from build123d import *

# Parameters (mm, degrees)
F0_R     = 11.65
F0_R_2   = 11
F1_DEPTH = 180
F3_DEPTH = 0.4
F4_COUNT = 8


with BuildPart() as f1:
    # F0 (on Front) → F1 (new body)
    with BuildSketch(Plane.XZ):
        Circle(F0_R)
        Circle(F0_R_2, mode=Mode.SUBTRACT)
    extrude(amount=F1_DEPTH)

    # F2 (on Top) → F3 (join, symmetric)
    with BuildSketch(Plane.XY):
        Polygon((-11.318761, -35.867412), (-11.318761, 0), (-23.984207, 0), (-23.984207, -22.375958), align=None)
    extrude(amount=F3_DEPTH, both=True)

    # F4: F1 ×8 about axis
    f4_axis = Axis((0, 0, 0), (0, 1, 0))


with BuildPart() as f1_1:
    add(f1.part)
    for i in range(1, F4_COUNT):
        add(f1.part.rotate(f4_axis, i * 360 / F4_COUNT))


solid = f1_1.part
Geometry: final body of the model. Coordinates: model frame, mm. A direction names the side the tool comes from. Give positions to 0.01 mm unless a question says otherwise; leave off trailing zeros. Write each loop counter-clockwise with the first axis right and the second up, starting at its lowest first coordinate (ties: lowest second). Pieces come first, ordered by that corner, then holes.
(1) Cut plane D-D, the plane x = 13.5. Return loops of the section in (y, z), then the cut area to 3 significant figures.
(2) Ray query, line 1 (Z direction, x = 0, y = -127); line 2 (X direction, y = -15, z = -12.5); line 3 (X direction, y = -10.5, z = -10). Return the intervals inside material, ascending.
(3) Cut plane A-A, the plane z = 14. Return loops of the section in (x, y).
(4) Mould query, pull axis Z, two halves, no side actions, for faces 1 (the flat face through (-12.94, -13.565, 12.374)), 2 (the flat face through (-12.374, -13.565, 12.94)), 3 (the flat face through (-0.006, -28.857, -17.9)). Classes: released by +Z, released by -Z, zero draft, split by the parting line, or undercut.
(5) First-contact query: P1, Ø5, axis at x = 7.5, y = -66, coming from the -Z side; P2, Ø2, axis at x = -9, y = -145, coming from the -Z side; P3, Ø17.5, axis at x = 0, z = 0, coming from the -Y side; P4, Ø10, axis at x = 11, y = -152.5, coming from the -Z side. Flat tips, straight axial feed; report the tip coordinate or a pass-through.
(6) Cut plane B-B, the plane x = -3. Return loops of the section in (y, z), then the cut area to 3 significant figures.
(7) Access query for faces 4 (the flat face through (18, -14, -0.4)), 5 (the flat face through (-12.374, -13.565, -12.94)), 6 (the flat face through (-12.94, -13.565, -12.374)), 7 (the flat face through (-0.4, -14, 18)). Directions: +Z, -Z, +X, -X, +Y, -Y. A direction counts if a zero-diameter tool reaches every point of the face in a straight line with its end or side. Return the directions, or none.
(8) Cut plane C-C, the plane y = -98. Return loops of the section in (x, z).
Values follow:
1. outline: (-33.54, -0.4) - (0, -0.4) - (0, 0.4) - (-33.54, 0.4) - close; (-28.01, -12.93) - (-27.16, -14.07) - (0, -14.07) - (0, -12.93) - close; (-28.01, 12.93) - (0, 12.93) - (0, 14.07) - (-27.16, 14.07) - close
1. area: 89.3 mm2
2. line 1: z = -11.65 to -11, 11 to 11.65
2. line 2: x = -13.07 to -11.93, -0.4 to 0.4, 11.93 to 13.07
2. line 3: x = -10.57 to -9.43, -5.98 to -4.58, 4.58 to 5.98, 9.43 to 10.57
3. outline: (-14.57, -26.41) - (-13.43, -27.26) - (-13.43, 0) - (-14.57, 0) - close; (-0.4, -33.01) - (0.4, -33.01) - (0.4, 0) - (-0.4, 0) - close; (13.43, -27.26) - (14.57, -26.41) - (14.57, 0) - (13.43, 0) - close
4. face 1: undercut
4. face 2: released by +Z
4. face 3: released by -Z
5. P1: stops at z = -10.52
5. P2: stops at z = -8.47
5. P3: passes through
5. P4: stops at z = -9.99
6. outline: (-180, -11.26) - (0, -11.26) - (0, -10.58) - (-180, -10.58) - close; (-180, 10.58) - (0, 10.58) - (0, 11.26) - (-180, 11.26) - close
6. area: 243 mm2
7. face 4: +X, +Y, -Y
7. face 5: -Z, +Y, -Y
7. face 6: -X, +Y, -Y
7. face 7: +Z, +Y, -Y
8. outline: circle Ø23.3 at (0, 0); hole circle Ø22 at (0, 0)
